```python
from build123d import *

# Parameters (mm, degrees)
F0_R     = 9.0940365485
F1_DEPTH = 25
F0_W     = 105.1995866001
F0_H     = 10
F0_W_2   = 33.5022409036
F0_W_3   = 33.7981618941
F2_DEPTH = 100
F4_DEPTH = 15


with BuildPart() as f1:
    # F0 (on Front) → F1 (new body)
    with BuildSketch(Plane.XZ):
        with BuildLine():
            Line((-138.9977484941, 0), (-33.7981618941, 0))
            Line((-33.7981618941, 0), (-33.7981618941, 20.7065277838))
            Line((-33.7981618941, 20.7065277838), (-12.7240127639, 20.7065277838))
            Line((-12.7240127639, 20.7065277838), (-69.619662283, 113.2961352765))
            ThreePointArc((-69.619662283, 113.2961352765), (-86.2499946989, 122.5961471904), (-102.8803271148, 113.2961352765))
            Line((-102.8803271148, 113.2961352765), (-159.7759766339, 20.7065277838))
            Line((-159.7759766339, 20.7065277838), (-138.9977484941, 20.7065277838))
            Line((-138.9977484941, 20.7065277838), (-138.9977484941, 0))
        make_face()
        with Locations((-86.2499946989, 103.0769153215)):
            Circle(F0_R, mode=Mode.SUBTRACT)
        Polygon((-172.4999893978, 0), (-138.9977484941, 0), (-138.9977484941, 20.7065277838), (-159.7759766339, 20.7065277838), align=None)
        Polygon((-33.7981618941, 0), (0, 0), (-12.7240127639, 20.7065277838), (-33.7981618941, 20.7065277838), align=None)
    extrude(amount=F1_DEPTH)

    # F0 (on Front) → F2 (join)
    with BuildSketch(Plane.XZ):
        with Locations((-86.3979551941, -5)):
            Rectangle(F0_W, F0_H)
        with Locations((-155.748868946, -5)):
            Rectangle(F0_W_2, F0_H)
        with Locations((-16.899080947, -5)):
            Rectangle(F0_W_3, F0_H)
    extrude(amount=F2_DEPTH)

    # F3 (on face) → F4 (join)
    with BuildSketch(Plane.XZ.offset(100)):
        Polygon((-140.0482910872, 21.6435156763), (-160.0482910872, 21.6435156763), (-172.4999893978, 0), (-172.4999893978, -10), (-140.0482910872, -10), align=None)
        Polygon((0, -10), (0, 0), (-12.8745967522, 21.6435156763), (-32.8745967522, 21.6435156763), (-32.8745967522, -10), align=None)
    extrude(amount=F4_DEPTH)


solid = f1.part
```
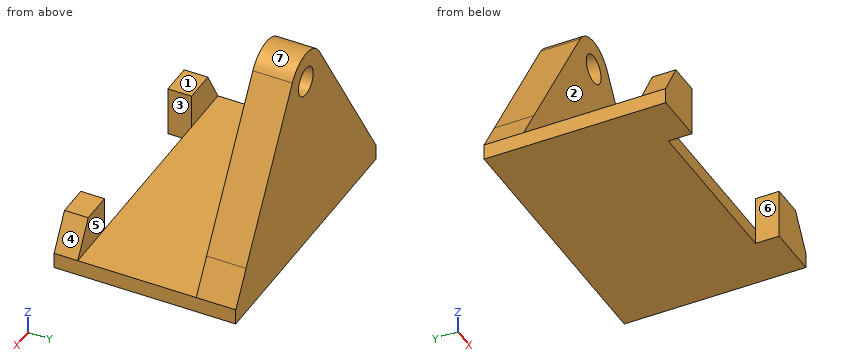
Source: CAD feature listing. Evaluate the final solid. Frame: model axes, mm. Face numbers are marked on the shaded views. A direction names the side the tool comes from. Coordinates: 2 decimals unless noted, no trailing zeros. Order: outer loops, then holes, each group sorted by start corner. A loop starts at its lowest first (then second) coordinate and runs counter-clockwise, first axis right, second up. Notation, with made-up numbers: (-25, -38) - (-10, -38) arc R21 ccw to (-10, -17) - close; hole circle Ø5 at (60, 14). An arc over 180 degrees is marked (long way). One line per item, written item: value.
1) Cut plane B-B on z = 109. Output: boundary loops of the cut face in (x, y).
Computed values:
outline: (-105.52, -25) - (-93.15, -25) - (-93.15, 0) - (-105.52, 0) - close; (-79.35, -25) - (-66.98, -25) - (-66.98, 0) - (-79.35, 0) - close
2) Cut plane C-C on x = -35.5. Output: boundary loops of the cut face in (y, z).
Computed values:
outline: (-100, -10) - (0, -10) - (0, 57.77) - (-25, 57.77) - (-25, 0) - (-100, 0) - close
3) Cut plane D-D on y = -17.5. Output: boundary loops of the cut face in (x, z), plus the area to 3 significant figures.
Computed values:
outline: (-172.5, -10) - (0, -10) - (0, 0) - (-69.62, 113.3) arc R19.52 ccw to (-102.88, 113.3) - (-172.5, 0) - close; hole circle Ø18.19 at (-86.25, 103.08)
area: 13,300 mm^2
4) Mould query, pull axis X, two halves, no side actions, for the marked faces 4, 5, 6 and 7. Classes: released by +X, released by -X, zero draft, split by the parting line, or undercut.
Computed values:
face 4: released by +X
face 5: zero draft
face 6: undercut
face 7: split by the parting line
5) Contact query for flat-ended pins moving along their axis: pin 1 (6 mm diameter, centred on x = -150.5, y = -55.5, fed in from +Z); pin 2 (5 mm diameter, centred on x = -25, z = 4, fed in from +Y); pin 3 (7.5 mm diameter, centred on x = -20, y = -107.5, fed in from +Z); pin 4 (11 mm diameter, centred on x = -75.5, z = -4.5, fed in from -Y). Output: stop coordinate, or through.
Computed values:
pin 1: stops at z = 0
pin 2: stops at y = 0
pin 3: stops at z = 21.64
pin 4: stops at y = -100
6) Ray query, line 1 (Y direction, x = -153, z = 18.5); line 2 (Z direction, x = -122, y = -52.5); line 3 (Y direction, x = -116.5, z = 22.5). Return the intervals inside material, ascending. Write a range as [from, to].
Computed values:
line 1: y = [-115, -100], [-25, 0]
line 2: z = [-10, 0]
line 3: y = [-25, 0]
7) Reachability of the marked faces 1, 2 and 3 from +Z, -Z, +X, -X, +Y, -Y: full face, straight path, thin tool, end or side. Return the list, or none.
Computed values:
face 1: +Z, +X, -X, -Y
face 2: +Z, +X, -X
face 3: +Z, -Z, -Y
8) Cut plane A-A on y = -106.5. Output: boundary loops of the cut face in (x, z).
Computed values:
outline: (-172.5, -10) - (-140.05, -10) - (-140.05, 21.64) - (-160.05, 21.64) - (-172.5, 0) - close; (-32.87, -10) - (0, -10) - (0, 0) - (-12.87, 21.64) - (-32.87, 21.64) - close
